Geometry: final body of the model. Coordinates: model frame, mm. A direction names the side the tool comes from. Coordinates: 2 decimals unless noted, no trailing zeros. Write each loop counter-clockwise with the first axis right and the second up, starting at its lowest first coordinate (ties: lowest second). Pieces come first, ordered by that corner, then holes. Notation, with made-up numbers: (29, -34) - (80, -34) arc R19 ccw to (80, 3) - close; hole circle Ø7 at (-13.5, 43.25). An arc over 180 degrees is marked (long way). Answer as a JSON object with one key per item and string values. Group by question number.
Item 1: Section A-A on x = 226. Return loops of the section in (y, z).
Item 2: First-contact query: pin 1 Ø12 at (y, z) = (171, 27.5) entering from -X; pin 2 Ø5 at (x, z) = (226, 107) entering from +Y; pin 3 Ø4 at (x, z) = (233, 19.5) entering from +Y. Flat tips, straight axial feed; report the tip coordinate or a pass-through.
Item 3: Section C-C on y = 181.5. Return loops of the section in (x, z), and give its area (3 significant figures).
Item 4: Set-up query: faces 1 (the flat face through (226.12, 188.62, 89.73)), 2 (the flat face through (223, 180, 0)), 3 (the flat face through (232.46, 170.24, 89.73)). Return all of +Z, -Z, +X, -X, +Y, -Y with unobstructed straight access to the full face (end or side cutting, diameter ignored); none if empty.
Item 5: Line query: line 1 along X through (y, z) = (186.25, 172); line 2 along X through (y, z) = (187.5, 141.5); line 3 along Y through (x, z) = (234, 51). Output: solid intervals per line, ascending. Write a range as from..to.
Item 6: Section B-B on z = 118. Return loops of the section in (x, y).
```python
from build123d import *

# Parameters (mm, degrees)
BOSS_EXTRUDE1_DEPTH = 182
BOSS_EXTRUDE2_DEPTH = 1


with BuildPart() as part:
    # Sketch1 → Boss-Extrude1 (new body)
    with BuildSketch(Plane.XY):
        with BuildLine():
            Line((229.466385633, 190.084774284), (234.388449239, 187.516604015))
            ThreePointArc((234.388449239, 187.516604015), (234.754582519, 187.177871366), (234.898637882, 186.70033452))
            Line((234.898637882, 186.70033452), (235.288181443, 172.459456354))
            ThreePointArc((235.288181443, 172.459456354), (235.168635365, 171.971488379), (234.816933894, 171.612726503))
            Line((234.816933894, 171.612726503), (230.041262707, 168.829103536))
            ThreePointArc((230.041262707, 168.829103536), (229.588841957, 168.700212112), (229.130051641, 168.80417836))
            Line((229.130051641, 168.80417836), (224.209349738, 171.322567703))
            ThreePointArc((224.209349738, 171.322567703), (223.838561786, 171.661566677), (223.692518777, 172.142269754))
            Line((223.692518777, 172.142269754), (223.302975216, 186.383147919))
            ThreePointArc((223.302975216, 186.383147919), (223.420709707, 186.867845739), (223.767778026, 187.226087233))
            Line((223.767778026, 187.226087233), (228.542087512, 190.059491125))
            ThreePointArc((228.542087512, 190.059491125), (229.000953, 190.192173087), (229.466385633, 190.084774284))
        make_face()
    extrude(amount=BOSS_EXTRUDE1_DEPTH)

    # Sketch5 → Boss-Extrude2 (add)
    with BuildSketch(Plane(origin=(0, 0, 0), x_dir=(-1, 0, 0), z_dir=(0, 0, -1))):
        with BuildLine():
            Line((-229.928971048, 190.971349003), (-234.851034654, 188.403178734))
            ThreePointArc((-234.851034654, 188.403178734), (-235.602571388, 187.707885402), (-235.898263974, 186.727678192))
            Line((-235.898263974, 186.727678192), (-236.287807535, 172.486800026))
            ThreePointArc((-236.287807535, 172.486800026), (-236.04242348, 171.485181553), (-235.320509935, 170.748775595))
            Line((-235.320509935, 170.748775595), (-230.544838748, 167.965152629))
            ThreePointArc((-230.544838748, 167.965152629), (-229.616185629, 167.70058602), (-228.67445814, 167.913990424))
            Line((-228.67445814, 167.913990424), (-223.753756236, 170.432379767))
            ThreePointArc((-223.753756236, 170.432379767), (-222.992665178, 171.128219765), (-222.692892685, 172.114926081))
            Line((-222.692892685, 172.114926081), (-222.303349124, 186.355804247))
            ThreePointArc((-222.303349124, 186.355804247), (-222.545014659, 187.350710298), (-223.257418051, 188.086048102))
            Line((-223.257418051, 188.086048102), (-228.031727536, 190.919451994))
            ThreePointArc((-228.031727536, 190.919451994), (-228.973609327, 191.191799179), (-229.928971048, 190.971349003))
        make_face()
    extrude(amount=BOSS_EXTRUDE2_DEPTH)


solid = part.part
```
Checks:
{
 "1": {"outline": "(169.28, -1) - (189.71, -1) - (189.71, 0) - (188.55, 0) - (188.55, 182) - (170.41, 182) - (170.41, 0) - (169.28, 0) - close"},
 "2": {"pin 1": "x = 223.56", "pin 2": "y = 190.03", "pin 3": "y = 189.28"},
 "3": {"outline": "(222.44, -1) - (236.04, -1) - (236.04, 0) - (235.04, 0) - (235.04, 182) - (223.44, 182) - (223.44, 0) - (222.44, 0) - close", "area": "2,130 mm^2"},
 "4": {"face 1": "+Z, -X, +Y", "face 2": "+Z", "face 3": "+Z, +X, -Y"},
 "5": {"line 1": "223.31..234.91", "line 2": "224.23..234.42", "line 3": "171.14..187.72"},
 "6": {"outline": "(223.3, 186.38) - (223.69, 172.14) arc R0.95 ccw to (224.21, 171.32) - (229.13, 168.8) arc R0.95 ccw to (230.04, 168.83) - (234.82, 171.61) arc R0.95 ccw to (235.29, 172.46) - (234.9, 186.7) arc R0.95 ccw to (234.39, 187.52) - (229.47, 190.08) arc R0.95 ccw to (228.54, 190.06) - (223.77, 187.23) arc R0.95 ccw to start"}
}
